The listing builds one solid part. Answer for the finished solid, in the listing's coordinates (mm). Give positions to 0.01 mm unless a question says otherwise; leave off trailing zeros. Loops run counter-clockwise (first coordinate to the right, second up) from the corner with the lowest first, then second, coordinate; pieces in that order, holes last. Notation, with made-up numbers: (50, 42.25) - (76, 42.25) arc R10 ccw to (76, 54.25) - close; hole circle Ø3 at (74.25, 69.5). An arc over 180 degrees is marked (long way). One line per item, written item: value. Start each with the question number.
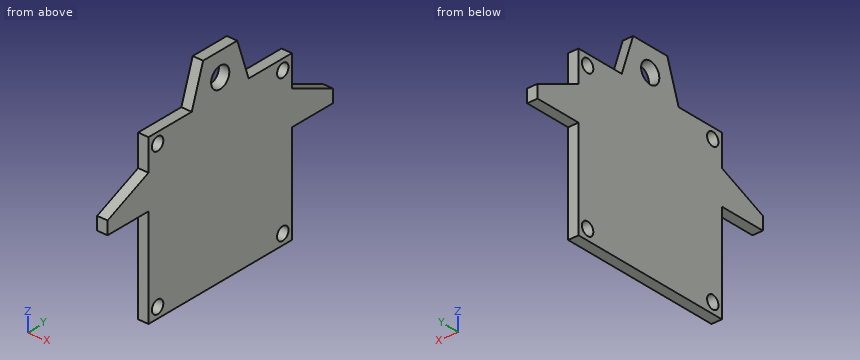
from build123d import *

# Parameters (mm, degrees)
F0_R     = 25
F0_R_2   = 40
F1_DEPTH = 40


with BuildPart() as f1:
    # F0 (on Right) → F1 (new body)
    with BuildSketch(Plane.YZ):
        Polygon((-125, 315), (-315, 315), (-315, 195), (-495, 115), (-495, 65), (-315, 65), (-315, -315), (-125, -315), (125, -315), (315, -315), (315, 65), (495, 65), (495, 115), (315, 195), (315, 315), (125, 315), (75, 465), (-75, 465), align=None)
        with Locations((-275, -275)):
            Circle(F0_R, mode=Mode.SUBTRACT)
        with Locations((275, -275)):
            Circle(F0_R, mode=Mode.SUBTRACT)
        with Locations((-275, 275)):
            Circle(F0_R, mode=Mode.SUBTRACT)
        with Locations((0, 375)):
            Circle(F0_R_2, mode=Mode.SUBTRACT)
        with Locations((275, 275)):
            Circle(F0_R, mode=Mode.SUBTRACT)
    extrude(amount=F1_DEPTH)


solid = f1.part
1. A cutting plane is placed at C-C (y = 275). Determine the outline of the cut face in (x, z), plus the area to 3 significant figures.
2. A cutting plane is placed at B-B (y = 0). Determine the outline of the cut face in (x, z), plus the area to 3 significant figures.
3. A cutting plane is placed at A-A (z = 375). Determine the outline of the cut face in (x, y).
4. Flat-ended cylindrical pins translate along their axes: pin 1 (2 mm diameter, centred on x = 22.5, z = 14.5, fed in from +Y); pin 2 (2 mm diameter, centred on x = 34.5, y = -371.5, fed in from +Z); pin 3 (12 mm diameter, centred on x = 7, y = -243.5, fed in from +Z). Find the tip coordinate at first contact, or state that the pin passes through.
5. Find the intervals of material crossed by L1, parallel to Z at x = 12, y = -275; L2, parallel to Y at x = 27, z = 276; L3, parallel to Z at x = 12, y = 0, in increasing order. Write a range as [from, to].
Results below:
1. outline: (0, -315) - (40, -315) - (40, -300) - (0, -300) - close; (0, -250) - (40, -250) - (40, 250) - (0, 250) - close; (0, 300) - (40, 300) - (40, 315) - (0, 315) - close
1. area: 21,200 mm^2
2. outline: (0, -315) - (40, -315) - (40, 335) - (0, 335) - close; (0, 415) - (40, 415) - (40, 465) - (0, 465) - close
2. area: 28,000 mm^2
3. outline: (0, -105) - (40, -105) - (40, -40) - (0, -40) - close; (0, 40) - (40, 40) - (40, 105) - (0, 105) - close
4. pin 1: stops at y = 315
4. pin 2: stops at z = 170.33
4. pin 3: stops at z = 315
5. L1: z = [-315, -300], [-250, 250], [300, 315]
5. L2: y = [-315, -299.98], [-250.02, 250.02], [299.98, 315]
5. L3: z = [-315, 335], [415, 465]
